Check sheet for the modelled part. Datum: model origin and axes. Units: mm. A direction names the side the tool comes from. Round coordinates to 2 decimals unless told otherwise and drop trailing zeros. Order: outer loops, then holes, each group sorted by start corner. A loop starts at its lowest first (then second) coordinate and runs counter-clockwise, first axis right, second up. Notation, with made-up numbers: (11.25, 52.5) -> (24.25, 52.5) arc R21 ccw to (24.25, 58.5) -> close; hole circle Ø11 at (41.25, 66.25). An arc over 180 degrees is marked (long way). Answer in a Markdown table with one row per item.
from build123d import *

# Parameters (mm, degrees)
SKETCH1_R           = 2.8
BOSS_EXTRUDE1_DEPTH = 5
FILLET1_R           = 2
BOSS_EXTRUDE2_DEPTH = 10
FILLET2_R           = 2
SKETCH3_W           = 8
SKETCH3_H           = 2
CUT_EXTRUDE1_DEPTH  = 4
SKETCH5_R           = 2
CUT_EXTRUDE2_DEPTH  = 5
SKETCH6_W           = 89.229867451
SKETCH6_H           = 38
CUT_EXTRUDE3_DEPTH  = 8.5
FILLET3_R           = 3


with BuildPart() as part:
    # Sketch1 → Boss-Extrude1 (new body)
    with BuildSketch(Plane.XY):
        with BuildLine():
            Line((0, 19), (120, 19))
            ThreePointArc((120, 19), (129.246621004, 16.598192673), (136.155494421, 10))
            Line((136.155494421, 10), (100, 10))
            Line((100, 10), (100, -10))
            Line((100, -10), (136.155494421, -10))
            ThreePointArc((136.155494421, -10), (129.246621004, -16.598192673), (120, -19))
            Line((120, -19), (0, -19))
            ThreePointArc((0, -19), (-19, 0), (0, 19))
        make_face()
        Circle(SKETCH1_R, mode=Mode.SUBTRACT)
        with BuildLine():
            Line((29.217733251, 11), (59.217733251, 11))
            ThreePointArc((59.217733251, 11), (70.217733251, 0), (59.217733251, -11))
            Line((59.217733251, -11), (29.217733251, -11))
            ThreePointArc((29.217733251, -11), (18.217733251, 0), (29.217733251, 11))
        make_face(mode=Mode.SUBTRACT)
    extrude(amount=BOSS_EXTRUDE1_DEPTH)

    # Fillet1
    fillet1_edges = [part.edges().sort_by_distance(p)[0] for p in [
        (136.155494421, 10, 2.5),
        (136.155494421, -10, 2.5),
    ]]
    fillet(fillet1_edges, radius=FILLET1_R)

    # Sketch2 → Boss-Extrude2 (add)
    with BuildSketch(Plane.XY.offset(5)):
        with BuildLine():
            Line((86, 19), (86, -19))
            Line((86, -19), (120, -19))
            ThreePointArc((120, -19), (127.286167394, -17.547414758), (133.458252765, -13.411764706))
            ThreePointArc((133.458252765, -13.411764706), (133.888690869, -11.233035011), (132.041594579, -10))
            Line((132.041594579, -10), (100, -10))
            Line((100, -10), (100, 10))
            Line((100, 10), (132.041594579, 10))
            ThreePointArc((132.041594579, 10), (133.888690869, 11.233035011), (133.458252765, 13.411764706))
            ThreePointArc((133.458252765, 13.411764706), (127.286167394, 17.547414758), (120, 19))
            Line((120, 19), (86, 19))
        make_face()
    extrude(amount=BOSS_EXTRUDE2_DEPTH)

    # Fillet2
    fillet2_edges = [part.edges().sort_by_distance(p)[0] for p in [
        (86, 0, 5),
        (86, 0, 15),
    ]]
    fillet(fillet2_edges, radius=FILLET2_R)

    # Sketch3 → Cut-Extrude1 (cut)
    with BuildSketch(Plane.XY.offset(15)):
        with Locations((96, 0)):
            Rectangle(SKETCH3_W, SKETCH3_H)
    extrude(amount=-CUT_EXTRUDE1_DEPTH, mode=Mode.SUBTRACT)

    # Sketch5 → Cut-Extrude2 (cut)
    with BuildSketch(Plane.XY.offset(5)):
        with Locations((79, 10)):
            Circle(SKETCH5_R)
        with Locations((79, -10)):
            Circle(SKETCH5_R)
    extrude(amount=-CUT_EXTRUDE2_DEPTH, mode=Mode.SUBTRACT)

    # Sketch6 → Cut-Extrude3 (cut)
    with BuildSketch(Plane(origin=(0, 0, 0), x_dir=(-1, 0, 0), z_dir=(0, 0, -1))):
        with Locations((-138.614933726, 0)):
            Rectangle(SKETCH6_W, SKETCH6_H)
    extrude(amount=-CUT_EXTRUDE3_DEPTH, mode=Mode.SUBTRACT)

    # Fillet3
    fillet3_edges = [part.edges().sort_by_distance(p)[0] for p in [
        (94, 0, 0),
        (94, 0, 8.5),
    ]]
    fillet(fillet3_edges, radius=FILLET3_R)


solid = part.part
Item 1: Mould release check, pull along Y, two halves, no side actions. Record for faces 6 (the flat face through (37, 13, 0)), 7 (the cylindrical face through (133.876, 11.203, 11.704)), 8 (the cylindrical face through (127.189, -17.587, 11.704)): pulls with the +Y half, pulls with the -Y half, needs draft (parallel to the pull), parting line crosses it, or undercut.
Result sheet:
| item | result |
|---|---|
| face 6 | needs draft |
| face 7 | undercut |
| face 8 | pulls with the -Y half |
Item 2: Set-up check for faces 1 (the flat face through (86, 0, 10)), 2 (the flat face through (116, -10, 12)), 3 (the flat face through (44, -11, 2)), 4 (the flat face through (96, 1, 13)), 5 (the flat face through (94, 0, 4)): record each of +Z, -Z, +X, -X, +Y, -Y from which the full face is reachable in a straight line by a thin tool's end or side.
Result sheet:
| item | result |
|---|---|
| face 1 | +Z, -X, +Y, -Y |
| face 2 | +Z, -Z, +X |
| face 3 | +Z, -Z |
| face 4 | +Z, +X |
| face 5 | -Z, +X, +Y, -Y |
Item 3: Depth check by flat-ended pin: P1, Ø5, axis at y = -1, z = 13, coming from the +X side; P2, Ø1.8, axis at y = 6, z = 10.5, coming from the -X side; P3, Ø3.5, axis at x = 79, y = 10, coming from the +Z side; P4, Ø1.6, axis at x = 95.5, y = 0.5, coming from the +Z side. Enter the tip coordinate at first touch or a pass-through.
Result sheet:
| item | result |
|---|---|
| P1 | stops at x = 100 |
| P2 | stops at x = 86 |
| P3 | passes through |
| P4 | stops at z = 15 |
Item 4: Cross-section at A-A (x = 79). Record the boundary of the cut face in (y, z).
Result sheet:
| item | result |
|---|---|
| outline | (-19, 0) -> (-12, 0) -> (-12, 5) -> (-19, 5) -> close; (-8, 0) -> (8, 0) -> (8, 5) -> (-8, 5) -> close; (12, 0) -> (19, 0) -> (19, 5) -> (12, 5) -> close |
Item 5: Cross-section at C-C (x = 7). Record the boundary of the cut face in (y, z), and give its area (3 significant figures).
Result sheet:
| item | result |
|---|---|
| outline | (-19, 0) -> (19, 0) -> (19, 5) -> (-19, 5) -> close |
| area | 190 mm^2 |
Item 6: Cross-section at B-B (y = 16.5). Record the boundary of the cut face in (x, z), and give its area (3 significant figures).
Result sheet:
| item | result |
|---|---|
| outline | (-9.42, 0) -> (91, 0) arc R3 ccw to (94, 3) -> (94, 5.5) arc R3 cw to (97, 8.5) -> (129.42, 8.5) -> (129.42, 15) -> (88, 15) arc R2 ccw to (86, 13) -> (86, 7) arc R2 cw to (84, 5) -> (-9.42, 5) -> close |
| area | 827 mm^2 |
Item 7: Scan lines: line 1 (Y direction, x = 79, z = 1.65); line 2 (X direction, y = -0.5, z = 4.5) (3 decimals); line 3 (Z direction, x = 36, y = -14.5). Record each from-to range of solid material in increasing order. Write a range as [from, to].
Result sheet:
| item | result |
|---|---|
| line 1 | y = [-19, -12], [-8, 8], [12, 19] |
| line 2 | x = [-18.993, -2.755], [2.755, 18.229], [70.206, 94] |
| line 3 | z = [0, 5] |
